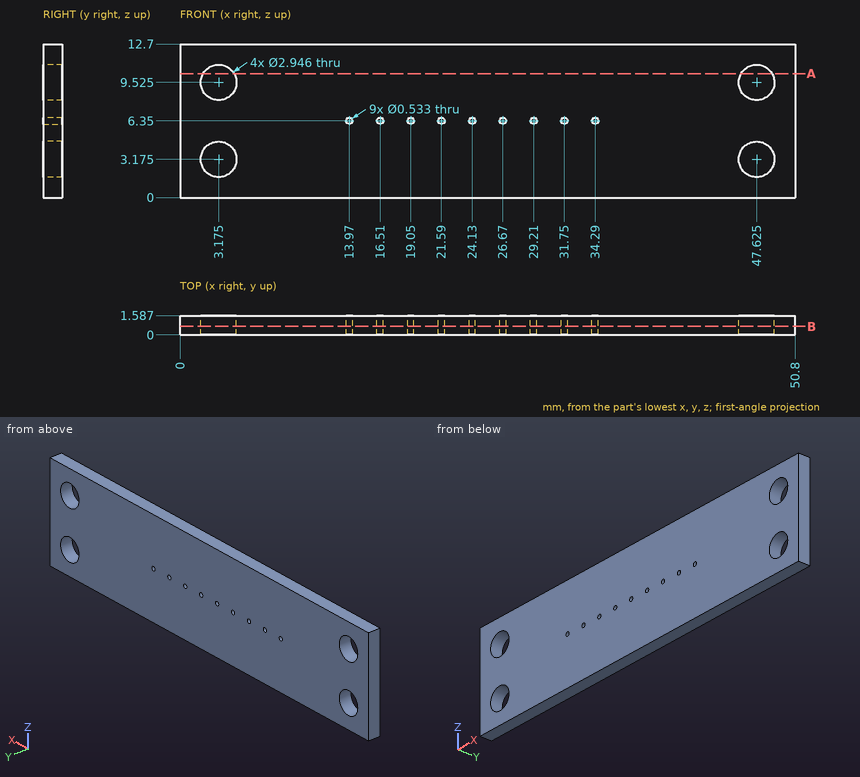
The figure shows three views and two pictorial views of one solid part (mm, origin at its lowest corner). Answer the questions. Round coordinates to 2 decimals unless told otherwise and drop trailing zeros. Order: outer loops, then holes, each group sorted by start corner. A loop starts at its lowest first (then second) coordinate and runs counter-clockwise, first axis right, second up. Notation, with made-up numbers: (67, -30.5) - (115, -30.5) arc R29 cw to (115, -10.5) - close; hole circle Ø5 at (49.5, 33.5). An arc over 180 degrees is marked (long way). Write item = value, one per line. Start each with the question number.
1) Section B-B, the plane y = 0.7 is taken. Count the separate pieces of the cut face and the enclosed holes in it, plus the area to 3 significant figures.
2) Section A-A, the plane z = 10.25 is taken. Write down the section's boundary in (x, y).
3) Straight lines are drawn through the part: L1, parallel to Z at x = 34.29, y = 0.75; L2, parallel to X at y = 0.45, z = 9.5; L3, parallel to X at y = 0.85, z = 8.5 (1 decimal). For each, find the intervals that lie inside material, in ascending order.
Results list:
q1.separate_pieces = 1
q1.enclosed_holes = 13
q1.area = 616 mm^2
q2.outline = (0, 0) - (1.89, 0) - (1.89, 1.59) - (0, 1.59) - close; (4.46, 0) - (46.34, 0) - (46.34, 1.59) - (4.46, 1.59) - close; (48.91, 0) - (50.8, 0) - (50.8, 1.59) - (48.91, 1.59) - close
q3.L1 = 0 to 6.08, 6.62 to 12.7
q3.L2 = 0 to 1.7, 4.65 to 46.15, 49.1 to 50.8
q3.L3 = 0 to 2.1, 4.2 to 46.6, 48.7 to 50.8
